Could you check a few things on this model? Use its own coordinates, in mm. Face numbers are marked on the shaded views. A direction names the side the tool comes from. Give positions to 0.01 mm unless a question says otherwise; leave off trailing zeros. Loops run counter-clockwise (first coordinate to the right, second up) from the corner with the lowest first, then second, coordinate; pieces in that order, holes last. Notation, with made-up numbers: (81.5, -10) -> (114.5, -10) arc R26 cw to (114.5, 12) -> close; hole circle Ø9 at (66.25, 10). An arc over 180 degrees is marked (long way). Put each result on its own line as item: value.
```python
from build123d import *

# Parameters (mm, degrees)
F0_R     = 9.5
F0_R_2   = 2.5
F1_DEPTH = 3
F2_SIZE  = 2.99999
F3_R     = 5.95
F3_R_2   = 2.5
F4_DEPTH = 17
F5_SIZE  = 1
F6_R     = 0.5


# Not quite as in the source:
# - a fillet or chamfer is up to 0.001 mm smaller than in the source, because OpenCascade refuses the exact size
# - a feature names something its author has since deleted; it is built from what else it names


with BuildPart() as f1:
    # F0 (on Top) → F1 (new body)
    with BuildSketch(Plane.XY):
        with Locations((-18.3589216322, 16.7421158403)):
            Circle(F0_R)
        with Locations((-18.3589216322, 16.7421158403)):
            Circle(F0_R_2, mode=Mode.SUBTRACT)
    extrude(amount=F1_DEPTH)

    # F2 (size 3 in the source; OpenCascade refuses exactly that, so slightly less here)
    f2_edges = [f1.edges().sort_by_distance(p)[0] for p in [
        (-20.858922, 16.742116, 3),
    ]]
    chamfer(f2_edges, length=F2_SIZE)

    # F3 (on face) → F4 (join)
    with BuildSketch(Plane(origin=(0, 0, 0), x_dir=(1, 0, 0), z_dir=(0, 0, -1))):
        with Locations((-18.3589216322, -16.7421158403)):
            Circle(F3_R)
        with Locations((-18.3589216322, -16.7421158403)):
            Circle(F3_R_2, mode=Mode.SUBTRACT)
    extrude(amount=F4_DEPTH)

    # F5
    f5_edges = [f1.edges().sort_by_distance(p)[0] for p in [
        (-24.308922, 16.742116, -17),
    ]]
    chamfer(f5_edges, length=F5_SIZE)

    # F6
    f6_edges = [f1.edges().sort_by_distance(p)[0] for p in [
        (-27.858922, 16.742116, 0),
        (-27.858922, 16.742116, 3),
        (-24.308922, 16.742116, 0),
    ]]
    fillet(f6_edges, radius=F6_R)


solid = f1.part
```
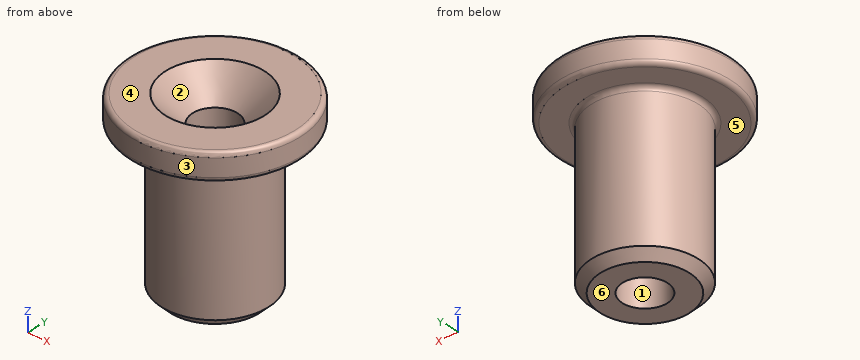
1. Thinking about a two-plate mould opening in X: for the marked faces 1, 2, 3 and 4, which applies, pulls with the +X half, pulls with the -X half, needs draft (parallel to the pull), parting line crosses it, or undercut?
Recorded:
face 1: undercut
face 2: undercut
face 3: parting line crosses it
face 4: needs draft
2. For the marked faces 5 and 6, which set-ups out of +Z, -Z, +X, -X, +Y, -Y let a thin tool reach every point of the face, with its end or its side?
Recorded:
face 5: -Z
face 6: -Z, +X, -X, +Y, -Y
3. If we section it at A-A (z = -5.25): List the corners of the cut face in (x, y) for me.
Recorded:
outline: circle Ø11.9 at (-18.36, 16.74); hole circle Ø5 at (-18.36, 16.74)
4. I need wall thicknesses on line 1 (Z direction, x = -23.75, y = 23.5); line 2 (Y direction, x = -19.75, z = -2.5); line 3 (Y direction, x = -16.5, z = -7.25). Which ranges of each line are inside material? Lowest first, please.
Recorded:
line 1: z = 0 to 3
line 2: y = 10.96 to 14.66, 18.82 to 22.53
line 3: y = 11.09 to 15.07, 18.41 to 22.39
5. I'm going to push flat-ended pins straight in: pin 1 (4 mm diameter, centred on y = 22.5, z = 1, fed in from +X); pin 2 (3 mm diameter, centred on x = -12, y = 11.5, fed in from -Z); pin 3 (3 mm diameter, centred on x = -19, y = 9.5, fed in from -Z). Where does each tip first touch, or does it pass through?
Recorded:
pin 1: stops at x = -9.63
pin 2: stops at z = 0
pin 3: stops at z = -16.18
6. If we section it at B-B (z = 1.5): List the corners of the cut face in (x, y) for me.
Recorded:
outline: circle Ø19 at (-18.36, 16.74); hole circle Ø8 at (-18.36, 16.74)
